Work out the finished part from the listing and answer in its coordinate system (mm). A direction names the side the tool comes from. Coordinates: 2 decimals unless noted, no trailing zeros. Order: outer loops, then holes, each group sorted by start corner. A loop starts at its lowest first (then second) coordinate and runs counter-clockwise, first axis right, second up. Notation, with made-up numbers: M 50.25,18.5 L 54.25,18.5 A15 ccw 54.25,35.5 Z; hole C 68.25,31 d2. An arc over 180 degrees is marked long. Use a Markdown table: item, result.
from build123d import *

# Parameters (mm, degrees)
BOSS_EXTRUDE1_DEPTH = 1.5
SKETCH2_R           = 2.75
BOSS_EXTRUDE2_DEPTH = 6
SKETCH3_W           = 1.1
SKETCH3_H           = 1.45
SKETCH3_W_2         = 1.45
SKETCH3_H_2         = 1.1
CUT_EXTRUDE1_DEPTH  = 6
CHAMFER1_SIZE       = 0.3
FILLET1_R           = 1
SKETCH4_R           = 1.25
BOSS_EXTRUDE3_DEPTH = 0.01
DOME1_FACE_RADIUS   = 1.25
DOME1_HEIGHT        = 1.25
DOME2_FACE_RADIUS   = 1.25
DOME2_HEIGHT        = 1.25
DOME3_FACE_RADIUS   = 1.25
DOME3_HEIGHT        = 1.25
FILLET3_R           = 0.2


with BuildPart() as part:
    # Sketch1 → Boss-Extrude1 (new body)
    with BuildSketch(Plane(origin=(0, 0, 0), x_dir=(1, 0, 0), z_dir=(0, 1, 0))):
        with BuildLine():
            Line((-7.324675649, 4.396717546), (4.675324351, 4.396717546))
            ThreePointArc((4.675324351, 4.396717546), (5.382431132, 4.103824327), (5.675324351, 3.396717546))
            Line((5.675324351, 3.396717546), (5.675324351, -8.603282454))
            ThreePointArc((5.675324351, -8.603282454), (5.382431132, -9.310389235), (4.675324351, -9.603282454))
            Line((4.675324351, -9.603282454), (-7.324675649, -9.603282454))
            ThreePointArc((-7.324675649, -9.603282454), (-8.03178243, -9.310389235), (-8.324675649, -8.603282454))
            Line((-8.324675649, -8.603282454), (-8.324675649, 3.396717546))
            ThreePointArc((-8.324675649, 3.396717546), (-8.03178243, 4.103824327), (-7.324675649, 4.396717546))
        make_face()
    extrude(amount=BOSS_EXTRUDE1_DEPTH)

    # Sketch2 → Boss-Extrude2 (add)
    with BuildSketch(Plane.XZ):
        with Locations(Location((-1.324675649, 2.603282454, 0), (0, 0, 270))):
            Circle(SKETCH2_R)
    extrude(amount=BOSS_EXTRUDE2_DEPTH)

    # Sketch3 → Cut-Extrude1 (cut)
    with BuildSketch(Plane.XZ.offset(6)):
        with Locations((-1.324675649, 3.878282454)):
            Rectangle(SKETCH3_W, SKETCH3_H)
        with Locations((-0.049675649, 2.603282454)):
            Rectangle(SKETCH3_W_2, SKETCH3_H_2)
        with Locations((-1.324675649, 2.603282454)):
            Rectangle(SKETCH3_W, SKETCH3_H_2)
        with Locations((-2.599675649, 2.603282454)):
            Rectangle(SKETCH3_W_2, SKETCH3_H_2)
        with Locations((-1.324675649, 1.328282454)):
            Rectangle(SKETCH3_W, SKETCH3_H)
    extrude(amount=-CUT_EXTRUDE1_DEPTH, mode=Mode.SUBTRACT)

    # Chamfer1
    chamfer1_edges = [part.edges().sort_by_distance(p)[0] for p in [
        (-0.774675649, -6, 3.878282454),
        (-0.049675649, -6, 3.153282454),
        (0.675324351, -6, 2.603282454),
        (-0.774675649, -6, 1.328282454),
        (-2.599675649, -6, 3.153282454),
        (-1.324675649, -6, 4.603282454),
        (-1.874675649, -6, 3.878282454),
        (-3.324675649, -6, 2.603282454),
        (-2.599675649, -6, 2.053282454),
        (-1.874675649, -6, 1.328282454),
        (-1.324675649, -6, 0.603282454),
        (-0.049675649, -6, 2.053282454),
    ]]
    chamfer(chamfer1_edges, length=CHAMFER1_SIZE)

    # Fillet1
    fillet1_edges = [part.edges().sort_by_distance(p)[0] for p in [
        (-1.324675649, 0, 5.353282454),
    ]]
    fillet(fillet1_edges, radius=FILLET1_R)

    # Sketch4 → Boss-Extrude3 (add)
    with BuildSketch(Plane(origin=(0, 1.5, 0), x_dir=(1, 0, 0), z_dir=(0, 1, 0))):
        with Locations(Location((-3.324675649, 1.396717546, 0), (0, 0, 90))):
            Circle(SKETCH4_R)
        with Locations(Location((-3.324675649, -2.603282454, 0), (0, 0, 90))):
            Circle(SKETCH4_R)
        with Locations(Location((0.675324351, 1.396717546, 0), (0, 0, 90))):
            Circle(SKETCH4_R)
    extrude(amount=BOSS_EXTRUDE3_DEPTH)

    # Dome1: a dome of height H over a round flat face of radius A is a cap of a sphere of radius (A * A + H * H) / (2 * H)
    dome1_r = (DOME1_FACE_RADIUS * DOME1_FACE_RADIUS + DOME1_HEIGHT * DOME1_HEIGHT) / (2 * DOME1_HEIGHT)
    dome1_base = Plane((-3.324675649, 1.51, -1.396717546), z_dir=(0, 1, 0))
    with Locations(dome1_base.offset(DOME1_HEIGHT - dome1_r)):
        dome1_ball = Sphere(dome1_r, mode=Mode.PRIVATE)
    add(split(dome1_ball, bisect_by=dome1_base, keep=Keep.TOP, mode=Mode.PRIVATE))

    # Dome2: a dome of height H over a round flat face of radius A is a cap of a sphere of radius (A * A + H * H) / (2 * H)
    dome2_r = (DOME2_FACE_RADIUS * DOME2_FACE_RADIUS + DOME2_HEIGHT * DOME2_HEIGHT) / (2 * DOME2_HEIGHT)
    dome2_base = Plane((0.675324351, 1.51, -1.396717546), z_dir=(0, 1, 0))
    with Locations(dome2_base.offset(DOME2_HEIGHT - dome2_r)):
        dome2_ball = Sphere(dome2_r, mode=Mode.PRIVATE)
    add(split(dome2_ball, bisect_by=dome2_base, keep=Keep.TOP, mode=Mode.PRIVATE))

    # Dome3: a dome of height H over a round flat face of radius A is a cap of a sphere of radius (A * A + H * H) / (2 * H)
    dome3_r = (DOME3_FACE_RADIUS * DOME3_FACE_RADIUS + DOME3_HEIGHT * DOME3_HEIGHT) / (2 * DOME3_HEIGHT)
    dome3_base = Plane((-3.324675649, 1.51, 2.603282454), z_dir=(0, 1, 0))
    with Locations(dome3_base.offset(DOME3_HEIGHT - dome3_r)):
        dome3_ball = Sphere(dome3_r, mode=Mode.PRIVATE)
    add(split(dome3_ball, bisect_by=dome3_base, keep=Keep.TOP, mode=Mode.PRIVATE))

    # Fillet3
    fillet3_edges = [part.edges().sort_by_distance(p)[0] for p in [
        (5.382431132, 1.5, 9.310389235),
        (-1.324675649, 0, 9.603282454),
        (-8.03178243, 0, 9.310389235),
        (5.675324351, 1.5, 2.603282454),
        (5.382431132, 1.5, -4.103824327),
        (-1.324675649, 1.5, -4.396717546),
        (-8.03178243, 1.5, -4.103824327),
        (-8.324675649, 1.5, 2.603282454),
        (-8.03178243, 1.5, 9.310389235),
        (-1.324675649, 1.5, 9.603282454),
        (-8.324675649, 0, 2.603282454),
        (-8.03178243, 0, -4.103824327),
        (-1.324675649, 0, -4.396717546),
        (5.382431132, 0, -4.103824327),
        (5.675324351, 0, 2.603282454),
        (5.382431132, 0, 9.310389235),
    ]]
    fillet(fillet3_edges, radius=FILLET3_R)


solid = part.part
(1) Determine the mould class of faces 1 (the flat face through (-0.775, -3, 1)), 2 (the cylindrical face through (5.375, 0.742, -4.112)), 3 (the cylindrical face through (-8.04, 0.742, -4.096)) for opening direction X: pulls with the +X half, pulls with the -X half, needs draft (parallel to the pull), parting line crosses it, or undercut.
Conclusion:
| item | result |
|---|---|
| face 1 | undercut |
| face 2 | pulls with the +X half |
| face 3 | pulls with the -X half |
(2) A cutting plane is placed at D-D (y = 1.75). Determine the outline of the cut face in (x, z), then the cut area to 3 significant figures.
Conclusion:
| item | result |
|---|---|
| outline | C -3.32,-1.4 d2.45; C -3.32,2.6 d2.45; C 0.68,-1.4 d2.45 |
| area | 14.2 mm2 |
(3) A cutting plane is placed at B-B (x = 4). Determine the outline of the cut face in (y, z), then the cut area to 3 significant figures.
Conclusion:
| item | result |
|---|---|
| outline | M 0,-4.2 A0.2 ccw 0.2,-4.4 L 1.3,-4.4 A0.2 ccw 1.5,-4.2 L 1.5,9.4 A0.2 ccw 1.3,9.6 L 0.2,9.6 A0.2 ccw 0,9.4 Z |
| area | 21.0 mm2 |
(4) Straight lines are drawn through the part: L1, parallel to Y at x = 5.25, z = 9; L2, parallel to X at y = -3.25, z = 4.25; L3, parallel to Z at x = -3.25, y = -3.5. For each, find the intervals that lie inside material, in ascending order.
Conclusion:
| item | result |
|---|---|
| L1 | 0 to 1.5 |
| L2 | -3.53 to -1.87, -0.77 to 0.88 |
| L3 | 0.64 to 2.05, 3.15 to 4.57 |
(5) Which of the six approach directions +Z, -Z, +X, -X, +Y, -Y give full straight-line access (tool end or side, diameter ignored) to faces 4 (the flat face through (0, -3, 2.053)), 5 (the cylindrical face through (5.39, 0.74, 9.3))?
Conclusion:
| item | result |
|---|---|
| face 4 | -Y |
| face 5 | +Z, +X, +Y, -Y |
(6) A cutting plane is placed at C-C (y = -1.25). Determine the outline of the cut face in (x, z), then the cut area to 3 significant figures.
Conclusion:
| item | result |
|---|---|
| outline | C -1.32,2.6 d5.5; hole M -3.32,2.05 L -1.87,2.05 L -1.87,0.6 L -0.77,0.6 L -0.77,2.05 L 0.68,2.05 L 0.68,3.15 L -0.77,3.15 L -0.77,4.6 L -1.87,4.6 L -1.87,3.15 L -3.32,3.15 Z |
| area | 16.2 mm2 |
(7) Given P1, Ø0.6, axis at x = -1, y = -2, coming from the -Z side; P2, Ø0.7, axis at y = -3, z = 4, coming from the -X side; P3, Ø1.2, axis at x = -0.5, z = 2.5, coming from the -Y side, each flat-ended and moving along its own axis, determine where each tip first touches the part or whether it passes through.
Conclusion:
| item | result |
|---|---|
| P1 | z = -0.15 |
| P2 | x = -3.87 |
| P3 | y = -5.85 |
(8) A cutting plane is placed at A-A (z = 8.25). Determine the outline of the cut face in (x, y), then the cut area to 3 significant figures.
Conclusion:
| item | result |
|---|---|
| outline | M -8.32,0.2 A0.2 ccw -8.12,0 L 5.48,0 A0.2 ccw 5.68,0.2 L 5.68,1.3 A0.2 ccw 5.48,1.5 L -8.12,1.5 A0.2 ccw -8.32,1.3 Z |
| area | 21.0 mm2 |
